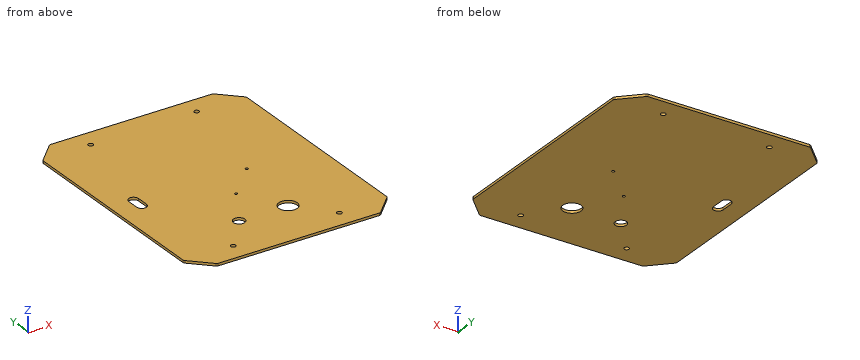
from build123d import *

# Parameters (mm, degrees)
BASE_DEPTH                     = 3
CONG_1_R                       = 3
ESQUISSE20_R                   = 3
PER_AGE_PROFIL_S_DEPTH         = 4
ESQUISSE21_R                   = 1.65
PER_AGE_LIDAR_DEPTH            = 4
ESQUISSE22_R                   = 11.25
PER_AGE_ARRET_D_URGENCE_DEPTH  = 4
ESQUISSE23_R                   = 7
PER_AGE_TIRETTE_DEPTH          = 4
PER_AGE_CABLE_MANAGEMENT_DEPTH = 4


with BuildPart() as part:
    # Esquisse1 → Base (new body)
    with BuildSketch(Plane.XY):
        Polygon((0, 0), (-200, 0), (-224.748737342, 24.748737342), (-224.748737342, 284.748737342), (-200, 309.497474683), (0, 309.497474683), (24.748737342, 284.748737342), (24.748737342, 24.748737342), align=None)
    extrude(amount=BASE_DEPTH)

    # Congé1
    cong_1_edges = [part.edges().sort_by_distance(p)[0] for p in [
        (0, 0, 1.5),
        (-200, 0, 1.5),
        (-224.748737342, 24.748737342, 1.5),
        (-224.748737342, 284.748737342, 1.5),
        (-200, 309.497474683, 1.5),
        (0, 309.497474683, 1.5),
        (24.748737342, 284.748737342, 1.5),
        (24.748737342, 24.748737342, 1.5),
    ]]
    fillet(cong_1_edges, radius=CONG_1_R)

    # Esquisse20 → Perçage Profilés (cut, through all)
    with BuildSketch(Plane(origin=(0, 0, 0), x_dir=(-1, 0, 0), z_dir=(0, 0, -1))):
        with Locations((35, 286.497474683)):
            Circle(ESQUISSE20_R)
        with Locations((165, 286.497474683)):
            Circle(ESQUISSE20_R)
        with Locations((165, 23)):
            Circle(ESQUISSE20_R)
        with Locations((35, 23)):
            Circle(ESQUISSE20_R)
    extrude(amount=-PER_AGE_PROFIL_S_DEPTH, mode=Mode.SUBTRACT)

    # Esquisse21 → Perçage Lidar (cut, through all)
    with BuildSketch(Plane(origin=(0, 0, 0), x_dir=(-1, 0, 0), z_dir=(0, 0, -1))):
        with Locations((61, 154.748737342)):
            Circle(ESQUISSE21_R)
        with Locations((100, 115.748737342)):
            Circle(ESQUISSE21_R)
    extrude(amount=-PER_AGE_LIDAR_DEPTH, mode=Mode.SUBTRACT)

    # Esquisse22 → Perçage Arret d'urgence (cut, through all)
    with BuildSketch(Plane(origin=(0, 0, 0), x_dir=(-1, 0, 0), z_dir=(0, 0, -1))):
        with Locations((70, 65)):
            Circle(ESQUISSE22_R)
    extrude(amount=-PER_AGE_ARRET_D_URGENCE_DEPTH, mode=Mode.SUBTRACT)

    # Esquisse23 → Perçage Tirette (cut, through all)
    with BuildSketch(Plane(origin=(0, 0, 0), x_dir=(-1, 0, 0), z_dir=(0, 0, -1))):
        with Locations((130, 65)):
            Circle(ESQUISSE23_R)
    extrude(amount=-PER_AGE_TIRETTE_DEPTH, mode=Mode.SUBTRACT)

    # Esquisse24 → Perçage Cable management (cut, through all)
    with BuildSketch(Plane(origin=(0, 0, 0), x_dir=(-1, 0, 0), z_dir=(0, 0, -1))):
        with BuildLine():
            Line((188.748737342, 147.248737342), (188.748737342, 162.248737342))
            ThreePointArc((188.748737342, 162.248737342), (194.748737342, 168.248737342), (200.748737342, 162.248737342))
            Line((200.748737342, 162.248737342), (200.748737342, 147.248737342))
            ThreePointArc((200.748737342, 147.248737342), (194.748737342, 141.248737342), (188.748737342, 147.248737342))
        make_face()
    extrude(amount=-PER_AGE_CABLE_MANAGEMENT_DEPTH, mode=Mode.SUBTRACT)


solid = part.part
Could you check a few things on this model? Use its own coordinates, in mm. Round coordinates to 2 decimals unless told otherwise and drop trailing zeros. Order: outer loops, then holes, each group sorted by start corner. A loop starts at its lowest first (then second) coordinate and runs counter-clockwise, first axis right, second up.
Q1. I'm going to push a flat-ended pin straight in: P1, Ø8, axis at x = -35, y = 23, coming from the -Z side. Where does the tip first touch, or does it pass through?
Geometry says:
P1: stops at z = 0
Q2. Please list where these lines run through material, in increasing order: probe 1 along Y at (x, z) = (-165, 1.75); probe 2 along X at (y, z) = (161.5, 1.5); probe 3 along X at (y, z) = (69, 1.9).
Geometry says:
probe 1: y = 0 to 20, 26 to 283.5, 289.5 to 309.5
probe 2: x = -224.75 to -200.75, -188.75 to 24.75
probe 3: x = -224.75 to -135.74, -124.26 to -80.51, -59.49 to 24.75
Q3. Imagine slicing it at C-C, the plane z = 1.7. State how many separate pieces and enclosed holes the cut face has, then the cut area to 3 significant figures.
Geometry says:
separate pieces: 1
enclosed holes: 9
area: 75,000 mm2
Q4. Imagine slicing it at D-D, the plane x = -207.5. List the corners of the cut face in (y, z) for me, then the cut area to 3 significant figures.
Geometry says:
outline: (7.5, 0) - (302, 0) - (302, 3) - (7.5, 3) - close
area: 883 mm2
Q5. Imagine slicing it at B-B, the plane x = -130. List the corners of the cut face in (y, z) for me.
Geometry says:
outline: (0, 0) - (58, 0) - (58, 3) - (0, 3) - close; (72, 0) - (309.5, 0) - (309.5, 3) - (72, 3) - close
Q6. Imagine slicing it at A-A, the plane y = 65. List the corners of the cut face in (x, z) for me.
Geometry says:
outline: (-224.75, 0) - (-137, 0) - (-137, 3) - (-224.75, 3) - close; (-123, 0) - (-81.25, 0) - (-81.25, 3) - (-123, 3) - close; (-58.75, 0) - (24.75, 0) - (24.75, 3) - (-58.75, 3) - close
